Can you work these out from the model? Positions are in its coordinate system, mm. A direction names the side the tool comes from. Give positions to 0.01 mm unless a question says otherwise; leave off trailing zeros. Write each loop counter-clockwise with the first axis right and the second up, starting at its lowest first coordinate (ties: lowest second). Pieces come first, ordered by that corner, then holes. Notation, with made-up numbers: (78.5, 28) -> (134.5, 28) arc R6 ccw to (134.5, 34) -> close; hole circle Ø7 at (9, 8). An arc over 180 degrees is marked (long way). One line per item, written item: value.
from build123d import *

# Parameters (mm, degrees)
SKETCH_1_R          = 36.5
EXTRUDE_1_DEPTH     = 6.5
CUT_EXTRUDE_START   = -4
CUT_EXTRUDE_2_DEPTH = 4
CUT_EXTRUDE_3_DEPTH = 4
SKETCH_6_R          = 1.5
CUT_EXTRUDE_5_DEPTH = 53.026435588
CUT_EXTRUDE_6_DEPTH = 2.2


with BuildPart() as part:
    # 草图1 → 凸台-拉伸1 (new body)
    with BuildSketch(Plane.XY):
        with Locations(Location((0, 0, 0), (0, 0, 180))):
            Circle(SKETCH_1_R)
    extrude(amount=EXTRUDE_1_DEPTH)

    # 草图3 → 切除-拉伸2 (cut)
    with BuildSketch(Plane.XY.offset(6.5).offset(CUT_EXTRUDE_START)):
        with BuildLine():
            Line((14, 33.708307581), (14, 26.532998323))
            ThreePointArc((14, 26.532998323), (21.213203436, 21.213203436), (26.532998323, 14))
            Line((26.532998323, 14), (33.708307581, 14))
            ThreePointArc((33.708307581, 14), (25.809397513, 25.809397513), (14, 33.708307581))
        make_face()
        with BuildLine():
            ThreePointArc((26.532998323, -14), (21.213203436, -21.213203436), (14, -26.532998323))
            Line((14, -26.532998323), (14, -33.708307581))
            ThreePointArc((14, -33.708307581), (25.809397513, -25.809397513), (33.708307581, -14))
            Line((33.708307581, -14), (26.532998323, -14))
        make_face()
        with BuildLine():
            Line((-14, -33.708307581), (-14, -26.532998323))
            ThreePointArc((-14, -26.532998323), (-21.213203436, -21.213203436), (-26.532998323, -14))
            Line((-26.532998323, -14), (-33.708307581, -14))
            ThreePointArc((-33.708307581, -14), (-25.809397513, -25.809397513), (-14, -33.708307581))
        make_face()
        with BuildLine():
            Line((-33.708307581, 14), (-26.532998323, 14))
            ThreePointArc((-26.532998323, 14), (-21.213203436, 21.213203436), (-14, 26.532998323))
            Line((-14, 26.532998323), (-14, 33.708307581))
            ThreePointArc((-14, 33.708307581), (-25.809397513, 25.809397513), (-33.708307581, 14))
        make_face()
    extrude(amount=CUT_EXTRUDE_2_DEPTH, mode=Mode.SUBTRACT)

    # 草图4 → 切除-拉伸3 (cut)
    with BuildSketch(Plane.XY.offset(6.5).offset(CUT_EXTRUDE_START)):
        with BuildLine():
            ThreePointArc((26.532998323, -14), (29.120353275, -7.211450974), (30, 0))
            ThreePointArc((30, 0), (29.120353275, 7.211450974), (26.532998323, 14))
            ThreePointArc((26.532998323, 14), (21.213203436, 21.213203436), (14, 26.532998323))
            ThreePointArc((14, 26.532998323), (0, 30), (-14, 26.532998323))
            ThreePointArc((-14, 26.532998323), (-21.213203436, 21.213203436), (-26.532998323, 14))
            ThreePointArc((-26.532998323, 14), (-30, 0), (-26.532998323, -14))
            ThreePointArc((-26.532998323, -14), (-21.213203436, -21.213203436), (-14, -26.532998323))
            ThreePointArc((-14, -26.532998323), (0, -30), (14, -26.532998323))
            ThreePointArc((14, -26.532998323), (21.213203436, -21.213203436), (26.532998323, -14))
        make_face()
    extrude(amount=CUT_EXTRUDE_3_DEPTH, mode=Mode.SUBTRACT)

    # 草图6 → 切除-拉伸5 (cut, through all)
    with BuildSketch(Plane(origin=(0, 0, 0), x_dir=(-1, 0, 0), z_dir=(0, 0, -1))):
        with Locations((32.9, 0)):
            Circle(SKETCH_6_R)
        with Locations((0, -32.9)):
            Circle(SKETCH_6_R)
        with Locations((0, 32.9)):
            Circle(SKETCH_6_R)
        with Locations((-32.9, 0)):
            Circle(SKETCH_6_R)
    extrude(amount=-CUT_EXTRUDE_5_DEPTH, mode=Mode.SUBTRACT)

    # 草图8 → 切除-拉伸6 (cut)
    with BuildSketch(Plane(origin=(0, 0, 0), x_dir=(-1, 0, 0), z_dir=(0, 0, -1))):
        Polygon((-29.998814897, -1.675), (-29.998814897, 1.675), (-32.9, 3.35), (-35.801185103, 1.675), (-35.801185103, -1.675), (-32.9, -3.35), align=None)
        Polygon((1.675, -35.801185103), (3.35, -32.9), (1.675, -29.998814897), (-1.675, -29.998814897), (-3.35, -32.9), (-1.675, -35.801185103), align=None)
        Polygon((35.801185103, -1.675), (35.801185103, 1.675), (32.9, 3.35), (29.998814897, 1.675), (29.998814897, -1.675), (32.9, -3.35), align=None)
        Polygon((1.675, 29.998814897), (3.35, 32.9), (1.675, 35.801185103), (-1.675, 35.801185103), (-3.35, 32.9), (-1.675, 29.998814897), align=None)
    extrude(amount=-CUT_EXTRUDE_6_DEPTH, mode=Mode.SUBTRACT)


solid = part.part
1) If we section it at D-D (x = -28): Write out the boundary of the cut face in (y, z), and give its area (3 significant figures).
Answer list:
outline: (-23.41, 0) -> (23.41, 0) -> (23.41, 2.5) -> (14, 2.5) -> (14, 6.5) -> (10.77, 6.5) -> (10.77, 2.5) -> (-10.77, 2.5) -> (-10.77, 6.5) -> (-14, 6.5) -> (-14, 2.5) -> (-23.41, 2.5) -> close
area: 143 mm^2
2) For faces 5 (the face through (-34.37, 2.5, 1.08)), 6 (the face through (30, 14, 4)), 7 (the face through (0, -30, 4)), 8 (the face through (14, 30, 4)), which set-ups out of +Z, -Z, +X, -X, +Y, -Y let a thin tool reach every point of the face, with its end or its side?
Answer list:
face 5: -Z
face 6: +Z, +X, -X, +Y
face 7: +Z
face 8: +Z, +X, +Y, -Y
3) If we section it at A-A (z = 4): Write out the boundary of the cut face in (x, y), and give its area (3 significant figures).
Answer list:
outline: (-33.71, -14) -> (-26.53, -14) arc R30 cw to (-26.53, 14) -> (-33.71, 14) arc R36.5 ccw to start; (-14, -33.71) arc R36.5 ccw to (14, -33.71) -> (14, -26.53) arc R30 cw to (-14, -26.53) -> close; (-14, 26.53) arc R30 cw to (14, 26.53) -> (14, 33.71) arc R36.5 ccw to (-14, 33.71) -> close; (26.53, -14) -> (33.71, -14) arc R36.5 ccw to (33.71, 14) -> (26.53, 14) arc R30 cw to start; hole circle Ø3 at (-32.9, 0); hole circle Ø3 at (0, -32.9); hole circle Ø3 at (0, 32.9); hole circle Ø3 at (32.9, 0)
area: 723 mm^2
4) I need wall thicknesses on L1, parallel to Y at x = 0, z = 3.5; L2, parallel to X at y = 33, z = 3; L3, parallel to X at y = 1, z = 5.75. Which ranges of each line are inside material? Lowest first, please.
Answer list:
L1: y = -36.5 to -34.4, -31.4 to -30, 30 to 31.4, 34.4 to 36.5
L2: x = -14 to -1.5, 1.5 to 14
L3: x = -36.49 to -34.02, -31.78 to -29.98, 29.98 to 31.78, 34.02 to 36.49
5) Will these pins go through, and if not, where does the flat tip stop? pin 1 (5 mm diameter, centred on x = 0, y = 32.9, fed in from -Z); pin 2 (1.5 mm diameter, centred on x = -5.5, z = 5.5, fed in from -Y); pin 3 (1.1 mm diameter, centred on x = -0.5, z = 0.5, fed in from +Y); pin 4 (8 mm diameter, centred on x = -9.5, y = -0.5, fed in from -Z).
Answer list:
pin 1: stops at z = 2.2
pin 2: stops at y = -36.19
pin 3: stops at y = 36.5
pin 4: stops at z = 0
6) If we section it at C-C (y = -13): Write out the boundary of the cut face in (x, z).
Answer list:
outline: (-34.11, 0) -> (34.11, 0) -> (34.11, 6.5) -> (27.04, 6.5) -> (27.04, 2.5) -> (-27.04, 2.5) -> (-27.04, 6.5) -> (-34.11, 6.5) -> close
7) If we section it at B-B (x = 0): Write out the boundary of the cut face in (y, z).
Answer list:
outline: (-36.5, 0) -> (-35.8, 0) -> (-35.8, 2.2) -> (-34.4, 2.2) -> (-34.4, 6.5) -> (-36.5, 6.5) -> close; (-31.4, 2.2) -> (-30, 2.2) -> (-30, 0) -> (30, 0) -> (30, 2.2) -> (31.4, 2.2) -> (31.4, 6.5) -> (30, 6.5) -> (30, 2.5) -> (-30, 2.5) -> (-30, 6.5) -> (-31.4, 6.5) -> close; (34.4, 2.2) -> (35.8, 2.2) -> (35.8, 0) -> (36.5, 0) -> (36.5, 6.5) -> (34.4, 6.5) -> close
8) We'd pull the mould along Y, two halves only. Please class faces 1 (the face through (-30, -14, 4)), 2 (the face through (0.2, 30.3, 6.5)), 3 (the face through (-35.801, 0, 1)), 4 (the face through (1.2, -33.8, 4.3)): released by +Y, released by -Y, zero draft, split by the parting line, or undercut.
Answer list:
face 1: released by -Y
face 2: zero draft
face 3: undercut
face 4: undercut
